```python
from build123d import *

# Parameters (mm, degrees)
SKETCH1_R           = 5
BOSS_EXTRUDE1_DEPTH = 20
BOSS_EXTRUDE2_DEPTH = 5
SKETCH3_W           = 10
SKETCH3_H           = 5
BOSS_EXTRUDE3_DEPTH = 20
SKETCH4_R           = 2.5
CUT_EXTRUDE1_DEPTH  = 52.720402164
FILLET1_RADIUS      = 5
FILLET1_LENGTH      = 5
FILLET2_RADIUS      = 5
FILLET2_LENGTH      = 5
FILLET4_R           = 5
FILLET5_R           = 5


with BuildPart() as part:
    # Sketch1 → Boss-Extrude1 (new body)
    with BuildSketch(Plane.XY):
        Circle(SKETCH1_R)
    extrude(amount=BOSS_EXTRUDE1_DEPTH)

    # Sketch2 → Boss-Extrude2 (add)
    with BuildSketch(Plane.XY.offset(20)):
        Polygon((-5, 0), (-5, 12.5), (5, 12.5), (5, -12.5), (-5, -12.5), align=None)
    extrude(amount=BOSS_EXTRUDE2_DEPTH)

    # Sketch3 → Boss-Extrude3 (add)
    with BuildSketch(Plane.XY.offset(25)):
        with Locations((0, 10)):
            Rectangle(SKETCH3_W, SKETCH3_H)
        with Locations((0, -10)):
            Rectangle(SKETCH3_W, SKETCH3_H)
    extrude(amount=BOSS_EXTRUDE3_DEPTH)

    # Sketch4 → Cut-Extrude1 (cut, through all)
    with BuildSketch(Plane(origin=(0, 12.5, 0), x_dir=(1, 0, 0), z_dir=(0, 1, 0))):
        with Locations(Location((0, -40, 0), (0, 0, 180))):
            Circle(SKETCH4_R)
    extrude(amount=-CUT_EXTRUDE1_DEPTH, mode=Mode.SUBTRACT)

    # Fillet1: full round fillet: the end face becomes a half cylinder, R = half its width
    fillet1_face = Plane((0, 10, 45), x_dir=(0, -1, 0), z_dir=(0, 0, 1))  # on the end face: x along it, z out of the body
    fillet1_slab = fillet1_face.offset(-FILLET1_RADIUS / 2) * Box(FILLET1_LENGTH, 2 * FILLET1_RADIUS, FILLET1_RADIUS, mode=Mode.PRIVATE)  # the body's end, R deep
    fillet1_round = Plane((0, 10, 40), x_dir=(0, 0, 1), z_dir=(0, -1, 0)) * Cylinder(FILLET1_RADIUS, FILLET1_LENGTH, mode=Mode.PRIVATE)  # its axis R under the face
    add(fillet1_slab - fillet1_round, mode=Mode.SUBTRACT)

    # Fillet2: full round fillet: the end face becomes a half cylinder, R = half its width
    fillet2_face = Plane((0, -10, 45), x_dir=(0, -1, 0), z_dir=(0, 0, 1))  # on the end face: x along it, z out of the body
    fillet2_slab = fillet2_face.offset(-FILLET2_RADIUS / 2) * Box(FILLET2_LENGTH, 2 * FILLET2_RADIUS, FILLET2_RADIUS, mode=Mode.PRIVATE)  # the body's end, R deep
    fillet2_round = Plane((0, -10, 40), x_dir=(0, 0, 1), z_dir=(0, -1, 0)) * Cylinder(FILLET2_RADIUS, FILLET2_LENGTH, mode=Mode.PRIVATE)  # its axis R under the face
    add(fillet2_slab - fillet2_round, mode=Mode.SUBTRACT)

    # Fillet4
    fillet4_edges = [part.edges().sort_by_distance(p)[0] for p in [
        (0, 12.5, 20),
    ]]
    fillet(fillet4_edges, radius=FILLET4_R)

    # Fillet5
    fillet5_edges = [part.edges().sort_by_distance(p)[0] for p in [
        (0, -12.5, 20),
    ]]
    fillet(fillet5_edges, radius=FILLET5_R)


solid = part.part
```
Verification items for the finished model (mm, model axes). A direction names the side the tool comes from. Coordinates: 2 decimals unless noted, no trailing zeros. Write each loop counter-clockwise with the first axis right and the second up, starting at its lowest first coordinate (ties: lowest second). Pieces come first, ordered by that corner, then holes. Notation, with made-up numbers: (68, -24) - (126, -24) arc R21 cw to (126, -7) - close; hole circle Ø8 at (10, 87). An arc over 180 degrees is marked (long way). One line per question, with ' | ' between items. Start each with the question number.
1. Section check A-A (x = 0). Enter the section's corners in (y, z), plus the area to 3 significant figures.
2. Section check D-D (x = -3.25). Enter the section's corners in (y, z), plus the area to 3 significant figures.
3. Draft check along X on faces 4 (the cylindrical face through (0, 10, 45)), 5 (the cylindrical face through (-0.07, -11, 21.43)), 6 (the cylindrical face through (0.54, -9.96, 37.56)). Enter one of: released by +X, released by -X, zero draft, split by the parting line, or undercut.
4. Access from +Z, -Z, +X, -X, +Y, -Y to the whole of each face (thin tool, end or side, straight path). Record for faces 1 (the flat face through (0, 7.5, 35)), 2 (the flat face through (0.1, 5.5, 20)), 3 (the cylindrical face through (-1.08, -4.88, 9.86)).
5. Section check B-B (y = 3). Enter the section's corners in (x, z).
6. Section check C-C (z = 12). Enter the section's corners in (x, y).
7. Material ranges on line 1 along Y through (x, z) = (4.5, 39); line 2 along Z through (x, y) = (-1, -4); line 3 along Z through (x, y) = (2.25, -6.5), recorded low to high.
8. Gauge pin test, flat ends, axial feed: P1, Ø1, axis at x = 2, z = 5, coming from the +Y side; P2, Ø6, axis at x = -3.5, z = 13, coming from the -Y side; P3, Ø1, axis at x = -1, z = 17, coming from the +Y side. Record the tip position at first contact, or that the pin passes through.
Computed values:
1) outline: (-12.5, 25) arc R5 ccw to (-7.5, 20) - (-5, 20) - (-5, 0) - (5, 0) - (5, 20) - (7.5, 20) arc R5 ccw to (12.5, 25) - (12.5, 37.5) - (7.5, 37.5) - (7.5, 25) - (-7.5, 25) - (-7.5, 37.5) - (-12.5, 37.5) - close; (-12.5, 42.5) - (-7.5, 42.5) - (-7.5, 45) - (-12.5, 45) - close; (7.5, 42.5) - (12.5, 42.5) - (12.5, 45) - (7.5, 45) - close | area: 464 mm²
2) outline: (-12.5, 25) arc R5 ccw to (-7.5, 20) - (-3.8, 20) - (-3.8, 0) - (3.8, 0) - (3.8, 20) - (7.5, 20) arc R5 ccw to (12.5, 25) - (12.5, 43.8) - (7.5, 43.8) - (7.5, 25) - (-7.5, 25) - (-7.5, 43.8) - (-12.5, 43.8) - close | area: 454 mm²
3) face 4: split by the parting line | face 5: zero draft | face 6: undercut
4) face 1: +Z, +X, -X | face 2: -Z, +Y | face 3: -Z
5) outline: (-5, 20) - (-4, 20) - (-4, 0) - (4, 0) - (4, 20) - (5, 20) - (5, 25) - (-5, 25) - close
6) outline: circle Ø10 at (0, 0)
7) line 1: -12.5 to -7.5, 7.5 to 12.5 | line 2: 0 to 25 | line 3: 20 to 25
8) P1: y = 4.77 | P2: y = -4.97 | P3: y = 4.97
